```python
from build123d import *

# Parameters (mm, degrees)
SKETCH1_W           = 100
SKETCH1_H           = 35
SKETCH1_R           = 2.35
SKETCH1_W_2         = 40.5
SKETCH1_H_2         = 20
BOSS_EXTRUDE1_DEPTH = 5.9
FILLET1_R           = 10
SKETCH3_W           = 10
SKETCH3_H           = 3.45
CUT_EXTRUDE2_DEPTH  = 10
CUT_EXTRUDE3_REACH  = 7.9
SKETCH4_R           = 2.05
CUT_EXTRUDE4_REACH  = 7.9
CUT_EXTRUDE5_START  = -5.9
SKETCH7_W           = 41.5
SKETCH7_H           = 21
CUT_EXTRUDE5_DEPTH  = 5.9


with BuildPart() as part:
    # Sketch1 → Boss-Extrude1 (new body)
    with BuildSketch(Plane(origin=(0, 0, 0), x_dir=(1, 0, 0), z_dir=(0, 1, 0))):
        Rectangle(SKETCH1_W, SKETCH1_H)
        with Locations((-4.8, 4.85)):
            Circle(SKETCH1_R, mode=Mode.SUBTRACT)
        with Locations((-4.8, -4.85)):
            Circle(SKETCH1_R, mode=Mode.SUBTRACT)
        with Locations((44.3, -4.85)):
            Circle(SKETCH1_R, mode=Mode.SUBTRACT)
        with Locations((44.3, 4.85)):
            Circle(SKETCH1_R, mode=Mode.SUBTRACT)
        with Locations((19.75, 0)):
            Rectangle(SKETCH1_W_2, SKETCH1_H_2, mode=Mode.SUBTRACT)
    extrude(amount=BOSS_EXTRUDE1_DEPTH)

    # Fillet1
    fillet1_edges = [part.edges().sort_by_distance(p)[0] for p in [
        (50, 2.95, 17.5),
        (-50, 2.95, 17.5),
        (-50, 2.95, -17.5),
        (50, 2.95, -17.5),
    ]]
    fillet(fillet1_edges, radius=FILLET1_R)

    # Sketch3 → Cut-Extrude2 (cut)
    with BuildSketch(Plane(origin=(0, 5.9, 0), x_dir=(1, 0, 0), z_dir=(0, 1, 0))):
        with Locations((-35, 15.775)):
            Rectangle(SKETCH3_W, SKETCH3_H)
        with Locations((-35, -15.775)):
            Rectangle(SKETCH3_W, SKETCH3_H)
    extrude(amount=-CUT_EXTRUDE2_DEPTH, mode=Mode.SUBTRACT)

    # Sketch4 → Cut-Extrude3 (cut, up to next)
    with BuildSketch(Plane(origin=(0, 5.9, 0), x_dir=(1, 0, 0), z_dir=(0, 1, 0)), mode=Mode.PRIVATE) as cut_extrude3_sk1:
        with Locations((-30, 14.05)):
            Circle(SKETCH4_R)
    cut_extrude3_tool1 = extrude(cut_extrude3_sk1.sketch, amount=-CUT_EXTRUDE3_REACH, mode=Mode.PRIVATE) & part.part
    add(cut_extrude3_tool1.solids().sort_by_distance((-30, 5.9, -14.05))[0], mode=Mode.SUBTRACT)
    # Sketch4 → Cut-Extrude3 (cut, up to next)
    with BuildSketch(Plane(origin=(0, 5.9, 0), x_dir=(1, 0, 0), z_dir=(0, 1, 0)), mode=Mode.PRIVATE) as cut_extrude3_sk2:
        with Locations((-40, 14.05)):
            Circle(SKETCH4_R)
    cut_extrude3_tool2 = extrude(cut_extrude3_sk2.sketch, amount=-CUT_EXTRUDE3_REACH, mode=Mode.PRIVATE) & part.part
    add(cut_extrude3_tool2.solids().sort_by_distance((-40, 5.9, -14.05))[0], mode=Mode.SUBTRACT)
    # Sketch4 → Cut-Extrude3 (cut, up to next)
    with BuildSketch(Plane(origin=(0, 5.9, 0), x_dir=(1, 0, 0), z_dir=(0, 1, 0)), mode=Mode.PRIVATE) as cut_extrude3_sk3:
        with Locations((-40, -14.05)):
            Circle(SKETCH4_R)
    cut_extrude3_tool3 = extrude(cut_extrude3_sk3.sketch, amount=-CUT_EXTRUDE3_REACH, mode=Mode.PRIVATE) & part.part
    add(cut_extrude3_tool3.solids().sort_by_distance((-40, 5.9, 14.05))[0], mode=Mode.SUBTRACT)
    # Sketch4 → Cut-Extrude3 (cut, up to next)
    with BuildSketch(Plane(origin=(0, 5.9, 0), x_dir=(1, 0, 0), z_dir=(0, 1, 0)), mode=Mode.PRIVATE) as cut_extrude3_sk4:
        with Locations((-30, -14.05)):
            Circle(SKETCH4_R)
    cut_extrude3_tool4 = extrude(cut_extrude3_sk4.sketch, amount=-CUT_EXTRUDE3_REACH, mode=Mode.PRIVATE) & part.part
    add(cut_extrude3_tool4.solids().sort_by_distance((-30, 5.9, 14.05))[0], mode=Mode.SUBTRACT)
    # Sketch4 → Cut-Extrude3 (cut, up to next)
    with BuildSketch(Plane(origin=(0, 5.9, 0), x_dir=(1, 0, 0), z_dir=(0, 1, 0)), mode=Mode.PRIVATE) as cut_extrude3_sk5:
        with Locations((-0.5, 10)):
            Circle(SKETCH4_R)
    cut_extrude3_tool5 = extrude(cut_extrude3_sk5.sketch, amount=-CUT_EXTRUDE3_REACH, mode=Mode.PRIVATE) & part.part
    add(cut_extrude3_tool5.solids().sort_by_distance((-0.5, 5.9, -10))[0], mode=Mode.SUBTRACT)
    # Sketch4 → Cut-Extrude3 (cut, up to next)
    with BuildSketch(Plane(origin=(0, 5.9, 0), x_dir=(1, 0, 0), z_dir=(0, 1, 0)), mode=Mode.PRIVATE) as cut_extrude3_sk6:
        with Locations((-0.5, -10)):
            Circle(SKETCH4_R)
    cut_extrude3_tool6 = extrude(cut_extrude3_sk6.sketch, amount=-CUT_EXTRUDE3_REACH, mode=Mode.PRIVATE) & part.part
    add(cut_extrude3_tool6.solids().sort_by_distance((-0.5, 5.9, 10))[0], mode=Mode.SUBTRACT)
    # Sketch4 → Cut-Extrude3 (cut, up to next)
    with BuildSketch(Plane(origin=(0, 5.9, 0), x_dir=(1, 0, 0), z_dir=(0, 1, 0)), mode=Mode.PRIVATE) as cut_extrude3_sk7:
        with Locations((40, -10)):
            Circle(SKETCH4_R)
    cut_extrude3_tool7 = extrude(cut_extrude3_sk7.sketch, amount=-CUT_EXTRUDE3_REACH, mode=Mode.PRIVATE) & part.part
    add(cut_extrude3_tool7.solids().sort_by_distance((40, 5.9, 10))[0], mode=Mode.SUBTRACT)
    # Sketch4 → Cut-Extrude3 (cut, up to next)
    with BuildSketch(Plane(origin=(0, 5.9, 0), x_dir=(1, 0, 0), z_dir=(0, 1, 0)), mode=Mode.PRIVATE) as cut_extrude3_sk8:
        with Locations((40, 10)):
            Circle(SKETCH4_R)
    cut_extrude3_tool8 = extrude(cut_extrude3_sk8.sketch, amount=-CUT_EXTRUDE3_REACH, mode=Mode.PRIVATE) & part.part
    add(cut_extrude3_tool8.solids().sort_by_distance((40, 5.9, -10))[0], mode=Mode.SUBTRACT)

    # Sketch6 → Cut-Extrude4 (cut, up to next)
    with BuildSketch(Plane(origin=(0, 5.9, 0), x_dir=(1, 0, 0), z_dir=(0, 1, 0)), mode=Mode.PRIVATE) as cut_extrude4_sk1:
        Polygon((40, -3.1), (40, 3.1), (40, 3.6), (45.5, 3.1), (45.5, -3.1), (40, -3.6), align=None)
    cut_extrude4_tool1 = extrude(cut_extrude4_sk1.sketch, amount=-CUT_EXTRUDE4_REACH, mode=Mode.PRIVATE) & part.part
    add(cut_extrude4_tool1.solids().sort_by_distance((42.681592, 5.9, 0))[0], mode=Mode.SUBTRACT)

    # Sketch7 → Cut-Extrude5 (cut)
    with BuildSketch(Plane(origin=(0, 5.9, 0), x_dir=(1, 0, 0), z_dir=(0, 1, 0)).offset(CUT_EXTRUDE5_START)):
        with Locations((19.75, 0)):
            Rectangle(SKETCH7_W, SKETCH7_H)
    extrude(amount=CUT_EXTRUDE5_DEPTH, mode=Mode.SUBTRACT)


solid = part.part
```
Geometry: final body of the model. Coordinates: model frame, mm. A direction names the side the tool comes from. Round coordinates to 2 decimals unless told otherwise and drop trailing zeros. Write each loop counter-clockwise with the first axis right and the second up, starting at its lowest first coordinate (ties: lowest second). Pieces come first, ordered by that corner, then holes.
Item 1: Section query D-D (z = -4.85). Return loops of the section in (x, y).
Item 2: Mould query, pull axis X, two halves, no side actions, for faces 1 (the face through (-12, 5.9, 0)), 2 (the face through (-47.15, 2.99, -14.49)), 3 (the face through (-1, 3, 0)). Classes: +X half, -X half, draft (parallel to the pull), parting line (faces both ways), or undercut.
Item 3: Set-up query: faces 4 (the face through (-50, 3, 0)), 5 (the face through (40.5, 3, -6)), 6 (the face through (-35, 3, -14.05)), 7 (the face through (5, 3, 17.5)), 8 (the face through (-35, 3, 14.05)). Return all of +Z, -Z, +X, -X, +Y, -Y with unobstructed straight access to the full face (end or side cutting, diameter ignored); none if empty.
Item 4: Material intervals for L1, parallel to X at y = 4.7, z = -4.85; L2, parallel to X at y = 1.6, z = 1; L3, parallel to Z at x = 0, y = 2.1, sorted ascending.
Item 5: Section query C-C (y = 3.45). Give the number of separate pieces and of enclosed holes in the cut face, plus the area to 3 significant figures.
Item 6: Section query B-B (x = -4.8). Return loops of the section in (y, z), plus the area to 3 significant figures.
Item 7: Section query A-A (z = -0.5). Return loops of the section in (x, y), plus the area to 3 significant figures.
Item 8: Pin query (flat end, axial travel): P1, Ø1.5, axis at y = 2, z = -17, coming from the -X side; P2, Ø3, axis at x = -4.8, z = 4.85, coming from the +Y side; P3, Ø1.8, axis at x = -35.5, y = 2, coming from the +Z side. Return the tip coordinate at first contact, or that it passes through.
Completed:
1. outline: (-50, 0) - (-7.15, 0) - (-7.15, 5.9) - (-50, 5.9) - close; (-2.45, 0) - (-1, 0) - (-1, 5.9) - (-2.45, 5.9) - close; (40.5, 0) - (41.95, 0) - (41.95, 5.9) - (40.5, 5.9) - close; (46.65, 0) - (50, 0) - (50, 5.9) - (46.65, 5.9) - close
2. face 1: draft
2. face 2: -X half
2. face 3: undercut
3. face 4: +Z, -Z, -X, +Y, -Y
3. face 5: +Y, -Y
3. face 6: -Z, +Y, -Y
3. face 7: +Z, +X, -X, +Y, -Y
3. face 8: +Z, +Y, -Y
4. L1: x = -50 to -7.15, -2.45 to -1, 40.5 to 41.95, 46.65 to 50
4. L2: x = -50 to -1, 45.5 to 50
4. L3: z = -17.5 to -11.99, 11.99 to 17.5
5. separate pieces: 1
5. enclosed holes: 3
5. area: 2,300 mm2
6. outline: (0, -17.5) - (5.9, -17.5) - (5.9, -7.2) - (0, -7.2) - close; (0, -2.5) - (5.9, -2.5) - (5.9, 2.5) - (0, 2.5) - close; (0, 7.2) - (5.9, 7.2) - (5.9, 17.5) - (0, 17.5) - close
6. area: 151 mm2
7. outline: (-50, 0) - (-1, 0) - (-1, 5.9) - (-50, 5.9) - close; (45.5, 0) - (50, 0) - (50, 5.9) - (45.5, 5.9) - close
7. area: 316 mm2
8. P1: stops at x = -44.84
8. P2: passes through
8. P3: stops at z = 14.05
